The listing builds one solid part. Answer for the finished solid, in the listing's coordinates (mm). Face numbers are marked on the shaded views. A direction names the side the tool comes from. Give positions to 0.01 mm unless a question says otherwise; leave off trailing zeros. Order: outer loops, then holes, each group sorted by start corner. A loop starts at its lowest first (then second) coordinate and runs counter-clockwise, first axis right, second up. Notation, with made-up numbers: (-22, 48.5) - (22, 48.5) arc R22 cw to (22, 67.5) - close; hole circle Ø5 at (57, -13.75). An arc over 180 degrees is marked (long way). Answer in a Markdown table with one row per item.
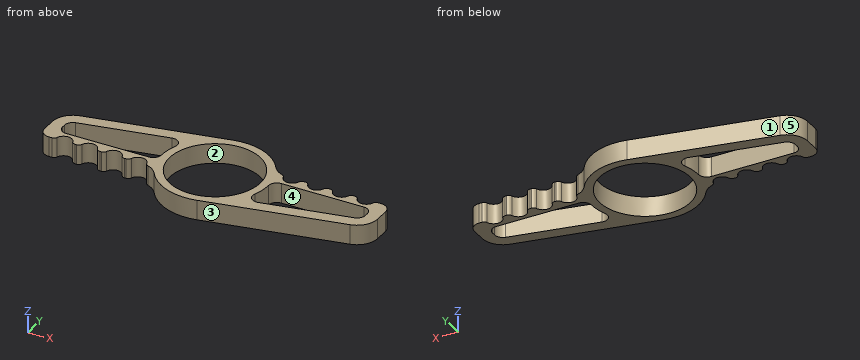
from build123d import *

# Parameters (mm, degrees)
F0_R     = 11
F1_DEPTH = 4.83


with BuildPart() as f1:
    # F0 (on Top) → F1 (new body)
    with BuildSketch(Plane.XY):
        with BuildLine():
            ThreePointArc((-36.01296, 5.824847), (-38.877164, 4.085682), (-40, 0.928531))
            Line((-40, 0.928531), (-40, -2.5))
            ThreePointArc((-40, -2.5), (-39.267767, -4.267767), (-37.5, -5))
            Line((-37.5, -5), (-36.828427, -5))
            ThreePointArc((-36.828427, -5), (-36.251077, -4.816497), (-35.885618, -4.333333))
            ThreePointArc((-35.885618, -4.333333), (-34, -3), (-32.114382, -4.333333))
            ThreePointArc((-32.114382, -4.333333), (-31.748923, -4.816497), (-31.171573, -5))
            Line((-31.171573, -5), (-30.828573, -5))
            ThreePointArc((-30.828573, -5), (-30.251193, -4.816476), (-29.88574, -4.333265))
            ThreePointArc((-29.88574, -4.333265), (-28.000073, -2.999794), (-26.114406, -4.333265))
            ThreePointArc((-26.114406, -4.333265), (-25.748953, -4.816476), (-25.171573, -5))
            Line((-25.171573, -5), (-24.828427, -5))
            ThreePointArc((-24.828427, -5), (-24.251077, -4.816497), (-23.885618, -4.333333))
            ThreePointArc((-23.885618, -4.333333), (-22, -3), (-20.114382, -4.333333))
            ThreePointArc((-20.114382, -4.333333), (-19.748923, -4.816497), (-19.171573, -5))
            Line((-19.171573, -5), (-18.828427, -5))
            ThreePointArc((-18.828427, -5), (-18.251077, -4.816497), (-17.885618, -4.333333))
            ThreePointArc((-17.885618, -4.333333), (-15.89445, -3.002787), (-14.054617, -4.535797))
            ThreePointArc((-14.054617, -4.535797), (-13.818534, -4.980014), (-13.396043, -5.253079))
            ThreePointArc((-13.396043, -5.253079), (-11.938126, -6.021537), (-10.809232, -7.222222))
            ThreePointArc((-10.809232, -7.222222), (-4.928987, -12.029343), (2.633697, -12.730422))
            Line((2.633697, -12.730422), (36.01296, -5.824847))
            ThreePointArc((36.01296, -5.824847), (38.877164, -4.085682), (40, -0.928531))
            Line((40, -0.928531), (40, 2.5))
            ThreePointArc((40, 2.5), (39.267767, 4.267767), (37.5, 5))
            Line((37.5, 5), (36.828427, 5))
            ThreePointArc((36.828427, 5), (36.251077, 4.816497), (35.885618, 4.333333))
            ThreePointArc((35.885618, 4.333333), (34, 3), (32.114382, 4.333333))
            ThreePointArc((32.114382, 4.333333), (31.748923, 4.816497), (31.171573, 5))
            Line((31.171573, 5), (30.828573, 5))
            ThreePointArc((30.828573, 5), (30.251193, 4.816476), (29.88574, 4.333265))
            ThreePointArc((29.88574, 4.333265), (28.000073, 2.999794), (26.114406, 4.333265))
            ThreePointArc((26.114406, 4.333265), (25.748953, 4.816476), (25.171573, 5))
            Line((25.171573, 5), (24.828427, 5))
            ThreePointArc((24.828427, 5), (24.251077, 4.816497), (23.885618, 4.333333))
            ThreePointArc((23.885618, 4.333333), (22, 3), (20.114382, 4.333333))
            ThreePointArc((20.114382, 4.333333), (19.748923, 4.816497), (19.171573, 5))
            Line((19.171573, 5), (18.828427, 5))
            ThreePointArc((18.828427, 5), (18.251077, 4.816497), (17.885618, 4.333333))
            ThreePointArc((17.885618, 4.333333), (15.89445, 3.002787), (14.054617, 4.535797))
            ThreePointArc((14.054617, 4.535797), (13.818534, 4.980014), (13.396043, 5.253079))
            ThreePointArc((13.396043, 5.253079), (11.938126, 6.021537), (10.809232, 7.222222))
            ThreePointArc((10.809232, 7.222222), (4.928987, 12.029343), (-2.633697, 12.730422))
            Line((-2.633697, 12.730422), (-36.01296, 5.824847))
        make_face()
        with BuildLine():
            ThreePointArc((14.451378, -7.222027), (12.527041, -6.564336), (12.173368, -4.5617))
            ThreePointArc((12.173368, -4.5617), (12.791673, -2.317996), (13, 0))
            ThreePointArc((13, 0), (13.585786, 1.414214), (15, 2))
            Line((15, 2), (35, 2))
            ThreePointArc((35, 2), (36.414214, 1.414214), (37, 0))
            Line((37, 0), (37, -0.928531))
            ThreePointArc((37, -0.928531), (36.550866, -2.191391), (35.405184, -2.887058))
            Line((35.405184, -2.887058), (14.451378, -7.222027))
        make_face(mode=Mode.SUBTRACT)
        with BuildLine():
            ThreePointArc((-14.451378, 7.222027), (-12.527041, 6.564336), (-12.173368, 4.5617))
            ThreePointArc((-12.173368, 4.5617), (-12.791673, 2.317996), (-13, 0))
            ThreePointArc((-13, 0), (-13.585786, -1.414214), (-15, -2))
            Line((-15, -2), (-35, -2))
            ThreePointArc((-35, -2), (-36.414214, -1.414214), (-37, 0))
            Line((-37, 0), (-37, 0.928531))
            ThreePointArc((-37, 0.928531), (-36.550866, 2.191391), (-35.405184, 2.887058))
            Line((-35.405184, 2.887058), (-14.451378, 7.222027))
        make_face(mode=Mode.SUBTRACT)
        Circle(F0_R, mode=Mode.SUBTRACT)
    extrude(amount=F1_DEPTH)


solid = f1.part
Item 1: Consider line 1 (Y direction, x = 0, z = 2.95); line 2 (X direction, y = 1, z = 3.7); line 3 (X direction, y = -1.25, z = 2.05). Determine where each line is inside the solid, lowest interval first.
Answer block:
| item | result |
|---|---|
| line 1 | -13 to -11, 11 to 13 |
| line 2 | -40 to -37, -12.96 to -10.95, 10.95 to 13.27, 36.73 to 40 |
| line 3 | -40 to -36.56, -13.44 to -10.93, 10.93 to 12.94, 36.97 to 39.99 |
Item 2: Find section A-A on x = 0. Write down the section's boundary in (y, z).
Answer block:
| item | result |
|---|---|
| outline | (-13, 0) - (-11, 0) - (-11, 4.83) - (-13, 4.83) - close; (11, 0) - (13, 0) - (13, 4.83) - (11, 4.83) - close |
Item 3: Determine the mould class of the marked faces 1, 2 and 3 for opening direction X: pulls with the +X half, pulls with the -X half, needs draft (parallel to the pull), parting line crosses it, or undercut.
Answer block:
| item | result |
|---|---|
| face 1 | pulls with the -X half |
| face 2 | undercut |
| face 3 | pulls with the +X half |
Item 4: Find section C-C on z = 2.95. Count the separate pieces of the cut face and the enclosed holes in it, then the cut area to 3 significant figures.
Answer block:
| item | result |
|---|---|
| separate pieces | 1 |
| enclosed holes | 3 |
| area | 491 mm² |
Item 5: Find section B-B on y = 9.25. Write down the section's boundary in (x, z), then the cut area to 3 significant figures.
Answer block:
| item | result |
|---|---|
| outline | (-19.46, 0) - (-5.95, 0) - (-5.95, 4.83) - (-19.46, 4.83) - close; (5.95, 0) - (9.13, 0) - (9.13, 4.83) - (5.95, 4.83) - close |
| area | 80.6 mm² |
Item 6: Each of these flat-tipped pins is pushed along its axis until it touches: P1, Ø1, axis at y = -10, z = 1.5, coming from the -X side; P2, Ø0.7, axis at x = 37, z = 3, coming from the +Y side; P3, Ø2, axis at y = 5, z = 3.5, coming from the -X side. Where does it stop, or does it pass through?
Answer block:
| item | result |
|---|---|
| P1 | x = -8.87 |
| P2 | y = 5 |
| P3 | x = -38.95 |
Item 7: Which of the six approach directions +Z, -Z, +X, -X, +Y, -Y give full straight-line access (tool end or side, diameter ignored) to the marked faces 4 and 5?
Answer block:
| item | result |
|---|---|
| face 4 | +Z, -Z |
| face 5 | +Z, -Z, -X, +Y |
